from build123d import *

# Parameters (mm, degrees)
F1_DEPTH = 3.175
F3_D     = 7.1374
F5_D     = 3.96875
F6_R     = 4.7752


with BuildPart() as f1:
    # F0 (on Front) → F1 (new body)
    with BuildSketch(Plane.XZ):
        with BuildLine():
            Line((12.7, -50.8), (12.7, 65.0875))
            ThreePointArc((12.7, 65.0875), (0, 77.7875), (-12.7, 65.0875))
            Line((-12.7, 65.0875), (-12.7, -65.0875))
            ThreePointArc((-12.7, -65.0875), (0, -77.7875), (12.7, -65.0875))
            Line((12.7, -65.0875), (12.7, -55.5625))
            Line((12.7, -55.5625), (0, -55.5625))
            Line((0, -55.5625), (0, -50.8))
            Line((0, -50.8), (12.7, -50.8))
        make_face()
    extrude(amount=F1_DEPTH)

    # F3 (through all)
    with Locations(Plane.XZ.offset(3.175)):
        with Locations((0, 65.0875)):
            Hole(F3_D / 2)

    # F5 (through all)
    with Locations(Plane.XZ.offset(3.175)):
        with Locations((-6.35, -41.275)):
            Hole(F5_D / 2)

    # F6
    f6_edges = [f1.edges().sort_by_distance(p)[0] for p in [
        (12.7, -1.5875, -55.5625),
        (12.7, -1.5875, -50.8),
    ]]
    fillet(f6_edges, radius=F6_R)


solid = f1.part
Geometry: final body of the model. Coordinates: model frame, mm. A direction names the side the tool comes from. Round coordinates to 2 decimals unless told otherwise and drop trailing zeros. Order: outer loops, then holes, each group sorted by start corner. A loop starts at its lowest first (then second) coordinate and runs counter-clockwise, first axis right, second up. Notation, with made-up numbers: (67, 34.25) -> (71, 34.25) arc R29 ccw to (71, 55.25) -> close; hole circle Ø8 at (67.5, 55.25). An arc over 180 degrees is marked (long way). Put each result on its own line as item: value. Start each with the question number.
Q1. Section C-C on x = -6.35. Return the cut outline in (y, z) (3 decimals), and give its area (3 significant figures).
Q2. Section A-A on x = 1.5. Return the cut outline in (y, z) (1 decimal).
Q3. Line query: probe 1 along Z at (x, y) = (2.5, -1.15); probe 2 along Z at (x, y) = (1.5, -0.55); probe 3 along Z at (x, y) = (5.25, -1.7). Output: solid intervals per line, ascending.
Q4. Reachability of faces 1 (the flat face through (12.7, -2, -63)), 2 (the flat face through (0, -2, -53)) from +Z, -Z, +X, -X, +Y, -Y: full face, straight path, thin tool, end or side. Return the list, or none.
Q5. Section B-B on y = -2.15. Give the number of separate pieces and of enclosed holes in the cut face, and give its area (3 significant figures).
Q6. Pull-direction query (X, two-part tool) for faces 3 (the flat face through (-12.7, -2, 1)), 4 (the cylindrical face through (-4.368, -1.565, -41.188)), 5 (the flat face through (4, -2, -50.8)); classes: +X half, -X half, draft (parallel to the pull), parting line (faces both ways), or undercut.
Ans:
1. outline: (-3.175, -76.086) -> (0, -76.086) -> (0, -43.259) -> (-3.175, -43.259) -> close; (-3.175, -39.291) -> (0, -39.291) -> (0, 76.086) -> (-3.175, 76.086) -> close
1. area: 471 mm2
2. outline: (-3.2, -77.7) -> (0, -77.7) -> (0, -55.6) -> (-3.2, -55.6) -> close; (-3.2, -50.8) -> (0, -50.8) -> (0, 61.8) -> (-3.2, 61.8) -> close; (-3.2, 68.3) -> (0, 68.3) -> (0, 77.7) -> (-3.2, 77.7) -> close
3. probe 1: z = -77.54 to -55.56, -50.8 to 62.54, 67.63 to 77.54
3. probe 2: z = -77.7 to -55.56, -50.8 to 61.85, 68.33 to 77.7
3. probe 3: z = -76.65 to -55.56, -50.8 to 76.65
4. face 1: +Z, -Z, +X, +Y, -Y
4. face 2: +X, +Y, -Y
5. separate pieces: 1
5. enclosed holes: 2
5. area: 3,690 mm2
6. face 3: -X half
6. face 4: undercut
6. face 5: draft
